Could you check a few things on this model? Use its own coordinates, in mm. A direction names the side the tool comes from. Give positions to 0.01 mm unless a question says otherwise; leave off trailing zeros. Order: outer loops, then holes, each group sorted by start corner. A loop starts at its lowest first (then second) coordinate and runs counter-clockwise, first axis right, second up.
(1) Imagine slicing it at B-B, the plane x = 0.1. Write out the boundary of the cut face in (y, z).
(2) On a 3-axis mill with a long thin cutter (end or side, diameter ignored), from which of +Z, -Z, +X, -X, +Y, -Y can I reach the whole of each face in a straight line? I mean faces 4 (the flat face through (-1, 3, 4.25)), 5 (the flat face through (-2.5, -2.2, 2.2)), 6 (the flat face through (-1, -3, 4.25)). Say none if no direction works.
(3) Will this pin go through, and if not, where does the flat tip stop? pin 1 (1 mm diameter, centred on x = -1, z = 1.5, fed in from -Y).
(4) If I drill on probe 1 along Z at (x, y) = (-0.2, -2.75); probe 2 along Y at (x, z) = (-0.75, 0.6); probe 3 along Y at (x, z) = (-1.9, 2.55), over which ranges is the centre line in solid material (lowest first)?
(5) Imagine slicing it at A-A, the plane y = 2.75. Write out the boundary of the cut face in (x, z), then the cut area to 3 significant figures.
(6) Imagine slicing it at D-D, the plane x = -1.9. Write out the boundary of the cut face in (y, z).
(7) Imagine slicing it at C-C, the plane z = 2.1. Write out the boundary of the cut face in (x, y).
(8) If we mould it in two halves opening along Y, with no side actions, what happens to faces 1 (the flat face through (-1, -2.5, 2)), 2 (the cylindrical face through (-0.5, 0, 2.2)), 3 (the flat face through (1, 0, 2))? For each: released by +Y, released by -Y, zero draft, split by the parting line, or undercut.
from build123d import *

# Parameters (mm, degrees)
BOSS_EXTRU_1_DEPTH      = 4.5
ESQUISSE2_W             = 4
ESQUISSE2_H             = 0.5
ENL_V_MAT_EXTRU_2_DEPTH = 7.68954408


with BuildPart() as part:
    # Esquisse1 → Boss.-Extru.1 (new body)
    with BuildSketch(Plane.XY):
        with BuildLine():
            Line((1, 3.5), (-2.5, 3.5))
            Line((-2.5, 3.5), (-2.5, 2))
            ThreePointArc((-2.5, 2), (-0.5, 0), (-2.5, -2))
            Line((-2.5, -2), (-2.5, -3.5))
            Line((-2.5, -3.5), (1, -3.5))
            Line((1, -3.5), (1, 3.5))
        make_face()
    extrude(amount=BOSS_EXTRU_1_DEPTH)

    # Esquisse2 → Enlèv. mat.-Extru.2 (cut, through all)
    with BuildSketch(Plane.ZY.offset(2.5)):
        Polygon((4.25, 3.5), (0, 3.5), (0, 3), (0.25, 3), (4.25, 3), align=None)
        with Locations((2.25, 2.75)):
            Rectangle(ESQUISSE2_W, ESQUISSE2_H)
        with Locations((2.25, -2.75)):
            Rectangle(ESQUISSE2_W, ESQUISSE2_H)
        Polygon((4.25, -3), (0.25, -3), (0, -3), (0, -3.5), (4.25, -3.5), align=None)
    extrude(amount=-ENL_V_MAT_EXTRU_2_DEPTH, mode=Mode.SUBTRACT)


solid = part.part
Answer block:
1. outline: (-3.5, 4.25) - (-2.5, 4.25) - (-2.5, 0.25) - (-3, 0.25) - (-3, 0) - (3, 0) - (3, 0.25) - (2.5, 0.25) - (2.5, 4.25) - (3.5, 4.25) - (3.5, 4.5) - (-3.5, 4.5) - close
2. face 4: +X, -X, +Y
2. face 5: +Z, -Z, -X, +Y, -Y
2. face 6: +X, -X, -Y
3. pin 1: stops at y = -2.5
4. probe 1: z = 0 to 0.25, 4.25 to 4.5
4. probe 2: y = -2.5 to -0.97, 0.97 to 2.5
4. probe 3: y = -2.5 to -1.91, 1.91 to 2.5
5. outline: (-2.5, 0) - (1, 0) - (1, 0.25) - (-2.5, 0.25) - close; (-2.5, 4.25) - (1, 4.25) - (1, 4.5) - (-2.5, 4.5) - close
5. area: 1.75 mm2
6. outline: (-3.5, 4.25) - (-2.5, 4.25) - (-2.5, 0.25) - (-3, 0.25) - (-3, 0) - (-1.91, 0) - (-1.91, 4.5) - (-3.5, 4.5) - close; (1.91, 0) - (3, 0) - (3, 0.25) - (2.5, 0.25) - (2.5, 4.25) - (3.5, 4.25) - (3.5, 4.5) - (1.91, 4.5) - close
7. outline: (-2.5, -2.5) - (1, -2.5) - (1, 2.5) - (-2.5, 2.5) - (-2.5, 2) arc R2 cw to (-2.5, -2) - close
8. face 1: released by -Y
8. face 2: undercut
8. face 3: zero draft
